Design review of the part built by this model. Coordinates are the model's own, in mm. A direction names the side the tool comes from. Round coordinates to 2 decimals unless told otherwise and drop trailing zeros. Loops run counter-clockwise (first coordinate to the right, second up) from the corner with the lowest first, then second, coordinate; pieces in that order, holes last. Notation, with made-up numbers: (48.25, 35.25) -> (84.25, 35.25) arc R31 ccw to (84.25, 63.25) -> close; hole circle Ø10 at (16.25, 64). An arc over 180 degrees is marked (long way). Answer as CSV lines item,"result". Start each with the question number.
Autodesk Inventor part; units mm, degrees
ref_plane "YZ Plane" through (0, 0, 0) normal (1, 0, 0) x (0, 1, 0)
ref_plane "XZ Plane" through (0, 0, 0) normal (0, 1, 0) x (-1, 0, 0)
ref_plane "XY Plane" through (0, 0, 0) normal (0, 0, 1) x (1, 0, 0)
sketch "Sketch1" plane through (0, 0, 0) normal (0, 1, 0) x (-1, 0, 0)
  line L0 (0, 9.3285) -> (174, 9.3285)
  line L1 (174, 9.3285) -> (174, 55.3285)
  line L2 (174, 55.3285) -> (0, 55.3285)
  line L3 (0, 55.3285) -> (0, 9.3285)
  circle A0 centre (12, 45.3285) radius 5
  circle A1 centre (162, 44.3285) radius 5
  circle A2 centre (162, 20.3285) radius 5
  circle A3 centre (12, 20.3285) radius 5
  point P0 (0, 0)
  dimension "d0" = 174
  dimension "d1" = 46
  dimension "d2" = 10
  dimension "d3" = 12
  dimension "d4" = 10
  dimension "d5" = 10
  dimension "d6" = 11
  dimension "d7" = 12
  dimension "d8" = 10
  dimension "d9" = 12
  dimension "d10" = 11
  dimension "d11" = 10
  dimension "d12" = 12
  dimension "d13" = 11
extrude "Extrusion1" add sketch "Sketch1" along normal blind 18
ref_plane "Work Plane1" through (-55, 0, 55.3285) normal (1, 0, 0) x (0, 0, -1)
sketch "Sketch2" plane through (-55, 0, 55.3285) normal (1, 0, 0) x (0, 0, -1)
  line L0 (46, 18) -> (0, 18)
  line L1 (0, 18) -> (0, 68)
  line L2 (46, 18) -> (46, 68)
  circle A0 centre (23, 68) radius 7
  arc A1 (46, 68) -> (0, 68) centre (23, 68) ccw
  point P0 (55.3285, 0)
  dimension "d17" = 50
  dimension "d18" = 50
  dimension "d20" = 14
extrude "Extrusion2" add sketch "Sketch2" against normal blind 14
ref_plane "Work Plane2" through (-119, 0, 9.3285) normal (-1, 0, 0) x (0, 0, 1)
sketch "Sketch3" plane through (-119, 0, 9.3285) normal (-1, 0, 0) x (0, 0, 1)
  line L0 (0, 0) -> (0, 18)
  line L1 (0, 18) -> (0, 68)
  circle A0 centre (23, 68) radius 7
  circle A1 centre (23, 68) radius 7
  line L2 (46, 0) -> (46, 18)
  line L3 (46, 18) -> (46, 68)
  line L4 (46, 18) -> (46, 68)
  arc A2 (46, 68) -> (0, 68) centre (23, 68) ccw
  line L5 (0, 18) -> (46, 18)
  point P0 (-9.3285, 0)
  dimension "d24" = 50
  dimension "d26" = 50
extrude "Extrusion3" add sketch "Sketch3" against normal blind 14
sketch "Sketch4" plane through (-105, 0, 9.3285) normal (1, 0, 0) x (0, 0, -1)
  line L0 (-46, 19.0772) -> (-46, 69.0772)
  circle A0 centre (-23, 68) radius 14
  point P0 (9.3285, 0)
  dimension "d31" = 28
extrude "Extrusion4" add sketch "Sketch4" along normal blind 2
sketch "Sketch5" plane through (-103, 68, 32.3285) normal (1, 0, 0) x (0, 0, -1)
  circle A0 centre (0, 0) radius 14
  circle A1 centre (0, 0) radius 7
  point P0 (32.3285, -68)
  dimension "d34" = 14
extrude "Extrusion5" cut sketch "Sketch5" against normal blind 50 contours A1
sketch "Sketch6" plane through (0, 18, 0) normal (0, 1, 0) x (1, 0, 0)
  line L0 (0.0001, -55.3285) -> (-23.9999, -55.3285)
  line L1 (-23.9999, -55.3285) -> (-23.9999, -9.3285)
  line L2 (0, -9.3285) -> (-174, -9.3285)
  line L3 (-55.709, -55.3285) -> (-23.9999, -55.3285)
  line L4 (-23.9999, -9.3285) -> (-55.709, -9.3285)
  line L5 (-55.709, -55.3285) -> (-55.709, -9.3285)
  line L6 (-174, -55.3285) -> (-150, -55.3285)
  line L7 (-150, -55.3285) -> (-150, -9.3285)
  line L8 (-150, -55.3285) -> (-118.7635, -55.3285)
  line L9 (-174, -55.3285) -> (0, -55.3285)
  line L10 (-118.7635, -9.3285) -> (-118.7635, -55.3285)
  line L11 (-118.7635, -9.3285) -> (-150, -9.3285)
  point P0 (0, 0)
  dimension "d37" = 24
  dimension "d38" = 24
extrude "Extrusion6" cut sketch "Sketch6" against normal blind 4 contours L3 L5 L2 L1 | L8 L7 L2 L10
sketch "Sketch7" plane through (-55, 0, 55.3285) normal (1, 0, 0) x (0, 0, -1)
  line L0 (0, 18) -> (0, 68)
  line L1 (23, 56) -> (28, 56)
  line L2 (23, 56) -> (18, 56)
  line L3 (18, 56) -> (18, 14)
  line L4 (0, 14) -> (46, 14)
  line L5 (28, 56) -> (28, 14)
  line L6 (18, 14) -> (28, 14)
  point P0 (55.3285, 0)
  dimension "d45" = 5
  dimension "d46" = 5
extrude "Extrusion7" add sketch "Sketch7" along normal blind 31
sketch "Sketch8" plane through (-55, 14, 37.3285) normal (0, 0, 1) x (1, 0, 0)
  line L0 (0, 4) -> (0, 42)
  line L1 (31, 42) -> (31, 0)
  line L2 (0, 42) -> (31, 0)
  line L3 (31, 0) -> (31, 42)
  line L4 (31, 42) -> (0, 42)
  point P0 (55, -14)
extrude "Extrusion8" cut sketch "Sketch8" against normal blind 31
sketch "Sketch9" plane through (-119, 0, 9.3285) normal (-1, 0, 0) x (0, 0, 1)
  line L0 (0, 18) -> (0, 14)
  line L1 (0, 18) -> (0, 68)
  line L2 (28, 56) -> (18, 56)
  line L3 (23, 56) -> (28, 56)
  line L4 (23, 56) -> (18, 56)
  line L5 (18, 56) -> (18, 14)
  line L6 (0, 14) -> (46, 14)
  line L7 (28, 14) -> (28, 56)
  line L8 (28, 14) -> (18, 14)
  point P0 (-9.3285, 0)
  dimension "d55" = 5
extrude "Extrusion9" add sketch "Sketch9" along normal blind 31
sketch "Sketch10" plane through (-119, 14, 27.3285) normal (0, 0, -1) x (-1, 0, 0)
  line L0 (0, 42) -> (31, 0)
  line L1 (31, 0) -> (31, 42)
  line L2 (31, 42) -> (0, 42)
  point P0 (-119, -14)
extrude "Extrusion10" cut sketch "Sketch10" against normal blind 31
sketch "Sketch11" plane through (-69, 0, 55.3285) normal (-1, 0, 0) x (0, 0, 1)
  circle A0 centre (-23, 68.0376) radius 14
  point P0 (-55.3285, 0)
  dimension "d60" = 28
extrude "Extrusion11" add sketch "Sketch11" along normal blind 2
sketch "Sketch12" plane through (-71, 68.0376, 32.3285) normal (-1, 0, 0) x (0, 0, 1)
  circle A0 centre (0, -0.0376) radius 7
  circle A1 centre (0, -0.0376) radius 7
  point P0 (-32.3285, -68.0376)
  dimension "d63" = 14
extrude "Extrusion12" cut sketch "Sketch12" against normal blind 50
properties part number "5 - Part1"
Q1. For pin 1 Ø1.2 at (y, z) = (16.5, 29.5) entering from +X; pin 2 Ø22.5 at (y, z) = (73.5, 26.5) entering from -X; pin 3 Ø25 at (x, y) = (-32, 34) entering from +Z; pin 4 Ø5 at (y, z) = (32.5, 49.5) entering from +X, all flat-tipped, find the tip position at first contact; note any pin that passes through.
Q2. To check wall thickness, follow probe 1 along X at (y, z) = (15, 51); probe 2 along Z at (x, y) = (-162, 14); probe 3 along X at (y, z) = (72, 53.5). State the ranges of each line that lie inside material, in increasing order. Write a range as from..to.
Q3. Machinability: for faces 5 (the flat face through (-86, 0, 33)), 6 (the flat face through (-127, 26, 27.328)), 7 (the flat face through (-131, 30, 37.328)), 8 (the flat face through (-12, 18, 33)), which of the approach directions +Z, -Z, +X, -X, +Y, -Y give a long, thin tool a straight path to every point of the face, cutting with its end or side? Answer none if there is none.
Q4. Add section B-B, the plane y = 22. Give the boundary of the cut face in (x, z).
Q5. Mouldability with a two-part tool opening along Y and no side actions: class faces 1 (the cylindrical face through (-104.014, 56.195, 24.802)), 2 (the flat face through (-134.283, 35.294, 32.258)), 3 (the flat face through (-55.709, 16, 33)), 4 (the flat face through (0, 9, 33)) as pulls with the +Y half, pulls with the -Y half, needs draft (parallel to the pull), parting line crosses it, or undercut.
Q6. Add section D-D, the plane z = 31.5. State how many separate pieces and enclosed holes the cut face has, and give its area (3 significant figures).
Q7. Add section A-A, the plane x = -61.5. Give the boundary of the cut face in (y, z).
Q8. Add section C-C, the plane x = -12. Give the boundary of the cut face in (y, z), and give its area (3 significant figures).
Worked answers:
1,pin 1,"stops at x = 0"
1,pin 2,"stops at x = -119"
1,pin 3,"stops at z = 37.33"
1,pin 4,"stops at x = -55"
2,probe 1,"x = -174..-150, -118.76..-55.71, -24..0"
2,probe 2,"z = 9.33..15.33, 25.33..39.33, 49.33..55.33"
2,probe 3,"x = -119..-105, -69..-55"
3,face 5,"+Z, -Z, +X, -X, -Y"
3,face 6,"-Z, +Y"
3,face 7,"+Z, +Y"
3,face 8,"+Z, -Z, +X, +Y"
4,outline,"(-144.1, 27.33) -> (-119, 27.33) -> (-119, 9.33) -> (-105, 9.33) -> (-105, 55.33) -> (-119, 55.33) -> (-119, 37.33) -> (-144.1, 37.33) -> close; (-69, 9.33) -> (-55, 9.33) -> (-55, 27.33) -> (-29.9, 27.33) -> (-29.9, 37.33) -> (-55, 37.33) -> (-55, 55.33) -> (-69, 55.33) -> close"
5,face 1,"undercut"
5,face 2,"pulls with the +Y half"
5,face 3,"undercut"
5,face 4,"needs draft"
6,separate pieces,"3"
6,enclosed holes,"2"
6,area,"5,890 mm^2"
7,outline,"(0, 9.33) -> (68, 9.33) arc R23 ccw to (68, 55.33) -> (0, 55.33) -> close; hole circle Ø14 at (68, 32.33)"
8,outline,"(0, 9.33) -> (18, 9.33) -> (18, 15.33) -> (0, 15.33) -> close; (0, 25.33) -> (18, 25.33) -> (18, 40.33) -> (0, 40.33) -> close; (0, 50.33) -> (18, 50.33) -> (18, 55.33) -> (0, 55.33) -> close"
8,area,"468 mm^2"
